Input: dimensioned drawing with shaded views. Units: mm. Origin: part minimum x, y, z. Round coordinates to 2 decimals unless told otherwise and drop trailing zeros. Loops run counter-clockwise (first coordinate to the right, second up) from the corner with the lowest first, then second, coordinate; pieces in that order, holes last. Notation, with made-up numbers: (15, 12.5) - (29, 12.5) arc R21 ccw to (29, 45.5) - close; hole circle Ø10 at (62.5, 22). An arc over 180 degrees is marked (long way). Answer as a JSON object with one key per item and string values. Group by question number.
Item 1: Line query: line 1 (X direction, y = 3.65, z = 40.24); line 2 (Z direction, x = 58.8, y = 1.7); line 3 (X direction, y = 2.35, z = 39). Output: solid intervals per line, ascending.
Item 2: Section C-C (x = 4). Return the cut outline in (y, z), plus the area to 3 significant figures.
Item 3: Section B-B (z = 40.24). Return the cut outline in (x, y).
Item 4: First-contact query: pin 1 (2 mm diameter, centred on x = 45.5, z = 39, fed in from -Y); pin 2 (2.5 mm diameter, centred on x = 47.5, y = 3, fed in from -Z); pin 3 (2 mm diameter, centred on y = 2, z = 13, fed in from +X); pin 4 (2 mm diameter, centred on y = 2, z = 12.5, fed in from +X). Flat tips, straight axial feed; report the tip coordinate or a pass-through.
Item 5: Section A-A (y = 1.25). Return the cut outline in (x, z).
Item 6: Section D-D (z = 4). Return the cut outline in (x, y).
Item 7: Draft query along Z for the marked faces 1, 2, 3 and 4. Return one class per face: released by +Z, released by -Z, zero draft, split by the parting line, or undercut.
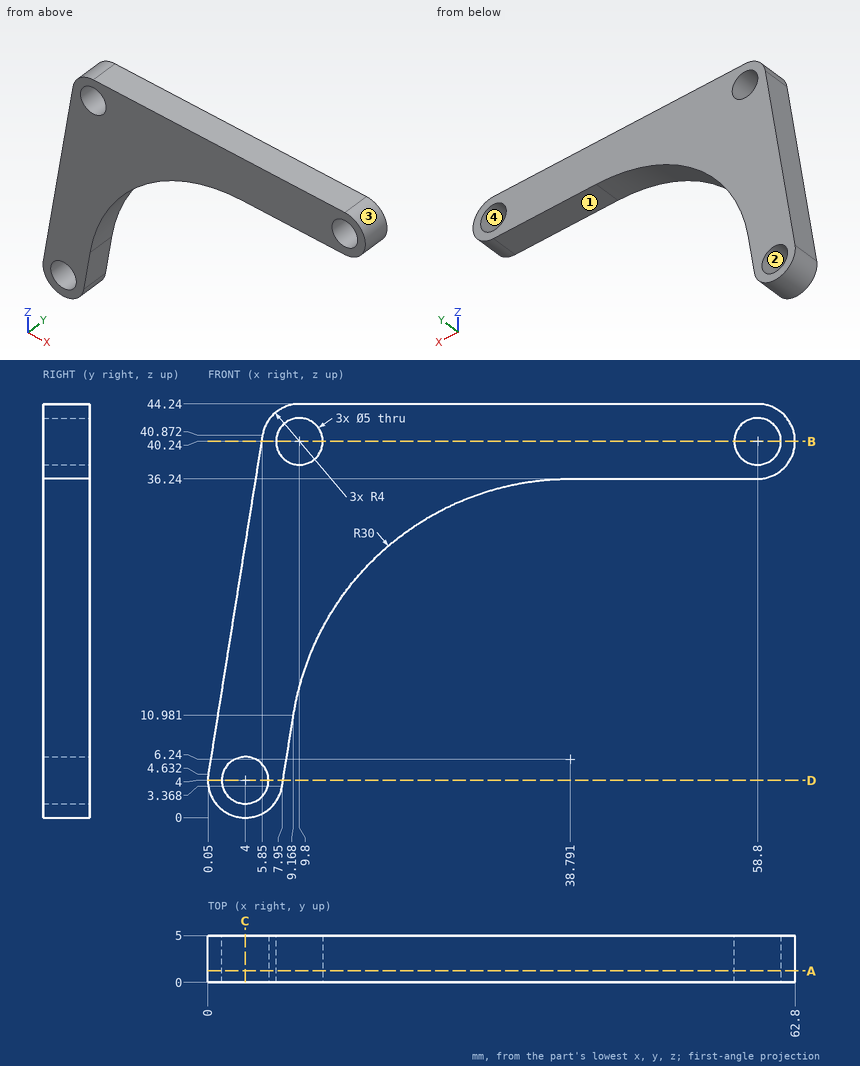
Values:
{
 "1": {"line 1": "x = 5.75 to 7.3, 12.3 to 56.3, 61.3 to 62.8", "line 2": "z = 36.24 to 37.74, 42.74 to 44.24", "line 3": "x = 5.55 to 7.63, 11.97 to 56.63, 60.97 to 62.6"},
 "2": {"outline": "(0, 0) - (5, 0) - (5, 1.5) - (0, 1.5) - close; (0, 6.5) - (5, 6.5) - (5, 29.31) - (0, 29.31) - close", "area": "122 mm^2"},
 "3": {"outline": "(5.75, 0) - (7.3, 0) - (7.3, 5) - (5.75, 5) - close; (12.3, 0) - (56.3, 0) - (56.3, 5) - (12.3, 5) - close; (61.3, 0) - (62.8, 0) - (62.8, 5) - (61.3, 5) - close"},
 "4": {"pin 1": "stops at y = 0", "pin 2": "stops at z = 36.24", "pin 3": "stops at x = 9.81", "pin 4": "stops at x = 9.68"},
 "5": {"outline": "(0.05, 4.63) arc R4 ccw to (7.95, 3.37) - (9.17, 10.98) arc R30 cw to (38.79, 36.24) - (58.8, 36.24) arc R4 ccw to (58.8, 44.24) - (9.8, 44.24) arc R4 ccw to (5.85, 40.87) - close; hole circle Ø5 at (4, 4); hole circle Ø5 at (9.8, 40.24); hole circle Ø5 at (58.8, 40.24)"},
 "6": {"outline": "(0, 0) - (1.5, 0) - (1.5, 5) - (0, 5) - close; (6.5, 0) - (8.05, 0) - (8.05, 5) - (6.5, 5) - close"},
 "7": {"face 1": "released by -Z", "face 2": "undercut", "face 3": "split by the parting line", "face 4": "undercut"}
}
